For this review, take the finished solid that the model builds, in its own axes (mm). Face numbers are marked on the shaded views. Round coordinates to 2 decimals unless told otherwise and drop trailing zeros. Order: outer loops, then holes, each group sorted by start corner. A loop starts at its lowest first (then second) coordinate and runs counter-clockwise, first axis right, second up.
from build123d import *


# Not quite as in the source:
# - a fillet or chamfer that OpenCascade refuses, or shapes differently, is made with other operations: its cross-section is extruded or revolved along the edge and cut away or added


with BuildPart() as f1:
    # F0 (on Front) → F1 (revolve)
    with BuildSketch(Plane.XZ):
        Polygon((2, 1.5050252532), (2, 0), (2, -2), (12, -2), (12, 16.28355698), (2, 16.28355698), (2, 14.28355698), (2, 12.8492424049), (3.8537319575, 10.9955104475), (7.3892658634, 7.4599765415), (7.3892658634, 6.8942911166), (3.1466251763, 2.6516504294), align=None)
    revolve(axis=Axis((15, 0, 2.570889245), (0, 0, 1)))

    # F2: chamfer of 0.5 on 2 edges, made by hand

    # F2_s1 → F2_t2 (revolve, cut)
    with BuildSketch(Plane.XZ):
        Polygon((2, 13.3492424049), (2.3535533906, 12.4956890143), (2, 12.8492424049), align=None)
    revolve(axis=Axis((15, 0, 12.8492424049), (0, 0, 1)), mode=Mode.SUBTRACT)

    # F2_s3 → F2_t4 (revolve, cut)
    with BuildSketch(Plane.XZ):
        Polygon((2.3535533906, 1.8585786438), (2, 1.0050252532), (2, 1.5050252532), align=None)
    revolve(axis=Axis((15, 0, 1.5050252532), (0, 0, 1)), mode=Mode.SUBTRACT)


solid = f1.part
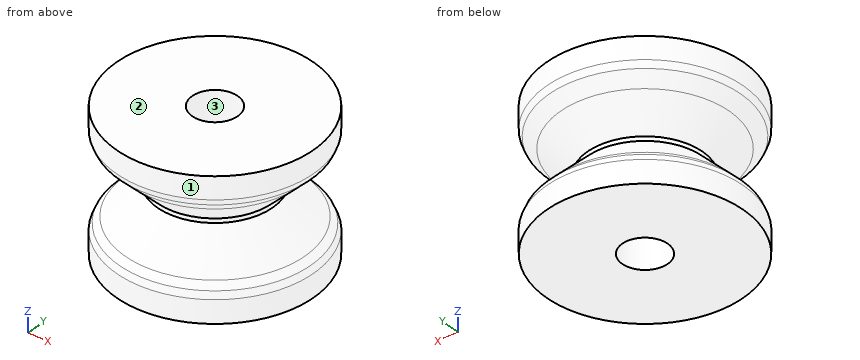
(1) Draft analysis for pull direction Y (two halves, no side actions). For the marked faces 1, 2 and 3, state which applies: pulls with the +Y half, pulls with the -Y half, needs draft (parallel to the pull), parting line crosses it, or undercut.
(2) Add section B-B on z = 5.5. Give the boundary of the cut face in (x, y).
(3) Wall thickness on L1, parallel to Y at x = 15, z = 7; L2, parallel to X at y = 0, z = 9.25; L3, parallel to X at y = 0, z = 2.25: over which ranges is each line inside the solid? List them lowest first.
(4) Add section A-A on z = 0.5. Give the boundary of the cut face in (x, y).
(5) Clearance check with flat-ended pins moving along their axes: P1, Ø5.5, axis at x = 15, y = 0, coming from the +Z side; P2, Ø10, axis at x = 9, z = 4.5, coming from the -Y side; P3, Ø4, axis at y = 9.5, z = 9, coming from the -X side; P4, Ø10, axis at y = 5, z = 1.5, coming from the +X side. State where each tip first meets the part, or that it passes through.
Here are the results:
1. face 1: parting line crosses it
1. face 2: needs draft
1. face 3: undercut
2. outline: circle Ø18.01 at (15, 0); hole circle Ø6 at (15, 0)
3. L1: y = -7.61 to -3, 3 to 7.61
3. L2: x = 5.6 to 12, 18 to 24.4
3. L3: x = 2.74 to 12, 18 to 27.26
4. outline: circle Ø26 at (15, 0); hole circle Ø6 at (15, 0)
5. P1: passes through
5. P2: stops at y = -12.77
5. P3: stops at x = 8.17
5. P4: stops at x = 28
